from build123d import *

# Parameters (mm, degrees)
F0_W     = 300
F0_H     = 24
F1_DEPTH = 100
F2_W     = 40
F2_H     = 15
F3_DEPTH = 300
F5_D     = 12


with BuildPart() as f1:
    # F0 (on Front) → F1 (new body, symmetric)
    with BuildSketch(Plane.XZ):
        with Locations((-5.195878, -20.055381)):
            Rectangle(F0_W, F0_H)
    extrude(amount=F1_DEPTH, both=True)

    # F2 (on face) → F3 (join)
    with BuildSketch(Plane.XY.offset(-8.055381)):
        with Locations((-35.195878, -92.5)):
            Rectangle(F2_W, F2_H)
        with Locations((-35.195878, 92.5)):
            Rectangle(F2_W, F2_H)
    extrude(amount=F3_DEPTH)

    # F5 (through all)
    with Locations(Plane.XZ.offset(100)):
        with Locations((-35.195878, 236.944619)):
            Hole(F5_D / 2)


solid = f1.part
For this review, take the finished solid that the model builds, in its own axes (mm). A direction names the side the tool comes from. Coordinates: 2 decimals unless noted, no trailing zeros. Order: outer loops, then holes, each group sorted by start corner. A loop starts at its lowest first (then second) coordinate and runs counter-clockwise, first axis right, second up. Notation, with made-up numbers: (70.25, 17) - (120.25, 17) arc R22 cw to (120.25, 53) - close; hole circle Ø6 at (26.5, 34.25). An arc over 180 degrees is marked (long way). Answer as CSV lines item,"result". Start each with the question number.
1) To check wall thickness, follow line 1 along Y through (x, z) = (-44.5, 34.5); line 2 along Z through (x, y) = (-100, -39). State the ranges of each line that lie inside material, in increasing order. Write a range as [from, to].
2) Add section B-B (x = 18). State the section outline as (y, z) points, then the cut area to 3 significant figures.
3) Insertion check: P1, Ø7.5, axis at y = 91.5, z = 105.5, coming from the -X side; P2, Ø16.5, axis at y = 94.5, z = 161.5, coming from the +X side; P3, Ø5, axis at x = 39, y = 52.5, coming from the +Z side. Each pin has a flat end and moves straight along its axis. Give the tip position at first contact, or say it passes through.
4) Machinability: for faces 1 (the flat face through (-55.196, -93, 140)), 2 (the flat face through (-15.196, -93, 140)), 3 (the flat face through (-35, 85, 140)), which of the approach directions +Z, -Z, +X, -X, +Y, -Y give a long, thin tool a straight path to every point of the face, cutting with its end or side? Answer none if there is none.
5) Add section A-A (z = -2). State the section outline as (x, y) points, then the cut area to 3 significant figures.
6) Add section C-C (y = 16.5). State the section outline as (x, z) points.
7) Draft analysis for pull direction Z (two halves, no side actions). For faces 4 (the cylindrical face through (-30.434, -92.395, 233.294)), 5 (the flat face through (-7, -1, -32.055)), 6 (the flat face through (-55.196, 92, 140)), 7 (the flat face through (-35, 93, 291.945)), state which applies: +Z half, -Z half, draft (parallel to the pull), parting line (faces both ways), or undercut.
Result:
1,line 1,"[-100, -85], [85, 100]"
1,line 2,"[-32.06, -8.06]"
2,outline,"(-100, -32.06) - (100, -32.06) - (100, -8.06) - (-100, -8.06) - close"
2,area,"4,800 mm^2"
3,P1,"x = -55.2"
3,P2,"x = -15.2"
3,P3,"z = -8.06"
4,face 1,"+Z, -X, +Y, -Y"
4,face 2,"+Z, +X, +Y, -Y"
4,face 3,"+Z, +X, -X"
5,outline,"(-55.2, -100) - (-15.2, -100) - (-15.2, -85) - (-55.2, -85) - close; (-55.2, 85) - (-15.2, 85) - (-15.2, 100) - (-55.2, 100) - close"
5,area,"1,200 mm^2"
6,outline,"(-155.2, -32.06) - (144.8, -32.06) - (144.8, -8.06) - (-155.2, -8.06) - close"
7,face 4,"undercut"
7,face 5,"-Z half"
7,face 6,"draft"
7,face 7,"+Z half"
